from build123d import *

# Parameters (mm, degrees)
SKETCH1_W           = 120
SKETCH1_H           = 70
BOSS_EXTRUDE1_DEPTH = 50
SKETCH4_W           = 116
SKETCH4_H           = 66
CUT_EXTRUDE1_DEPTH  = 48
SKETCH5_R           = 4
SKETCH5_R_2         = 2.125
SKETCH5_R_3         = 3.805710372
BOSS_EXTRUDE2_DEPTH = 48
SKETCH7_R           = 4
SKETCH7_R_2         = 2.125
BOSS_EXTRUDE3_DEPTH = 8
SKETCH9_R           = 3
CUT_EXTRUDE2_DEPTH  = 3
CUT_EXTRUDE3_START  = -3
SKETCH10_R          = 3
CUT_EXTRUDE3_DEPTH  = 3


with BuildPart() as part:
    # Sketch1 → Boss-Extrude1 (new body)
    with BuildSketch(Plane(origin=(0, 0, 0), x_dir=(1, 0, 0), z_dir=(0, 1, 0))):
        Rectangle(SKETCH1_W, SKETCH1_H)
    extrude(amount=BOSS_EXTRUDE1_DEPTH)

    # Sketch4 → Cut-Extrude1 (cut)
    with BuildSketch(Plane(origin=(0, 50, 0), x_dir=(1, 0, 0), z_dir=(0, 1, 0))):
        Rectangle(SKETCH4_W, SKETCH4_H)
    extrude(amount=-CUT_EXTRUDE1_DEPTH, mode=Mode.SUBTRACT)

    # Sketch5 → Boss-Extrude2 (add)
    # profile 1 of 4: a face of its own
    with BuildSketch(Plane(origin=(0, 2, 0), x_dir=(1, 0, 0), z_dir=(0, 1, 0))):
        with Locations(Location((-53.5, 28.5, 0), (0, 0, 270))):
            Circle(SKETCH5_R)
        with Locations(Location((-53.5, 28.5, 0), (0, 0, 270))):
            Circle(SKETCH5_R_2, mode=Mode.SUBTRACT)
    # profile 2 of 4: a face of its own
    with BuildSketch(Plane(origin=(0, 2, 0), x_dir=(1, 0, 0), z_dir=(0, 1, 0))):
        with Locations(Location((-53.5, -28.5, 0), (0, 0, 270))):
            Circle(SKETCH5_R_3)
        with Locations(Location((-53.5, -28.5, 0), (0, 0, 270))):
            Circle(SKETCH5_R_2, mode=Mode.SUBTRACT)
    # profile 3 of 4: a face of its own
    with BuildSketch(Plane(origin=(0, 2, 0), x_dir=(1, 0, 0), z_dir=(0, 1, 0))):
        with Locations(Location((53.5, -28.5, 0), (0, 0, 270))):
            Circle(SKETCH5_R)
        with Locations(Location((53.5, -28.5, 0), (0, 0, 270))):
            Circle(SKETCH5_R_2, mode=Mode.SUBTRACT)
    # profile 4 of 4: a face of its own
    with BuildSketch(Plane(origin=(0, 2, 0), x_dir=(1, 0, 0), z_dir=(0, 1, 0))):
        with Locations(Location((53.5, 28.5, 0), (0, 0, 270))):
            Circle(SKETCH5_R)
        with Locations(Location((53.5, 28.5, 0), (0, 0, 270))):
            Circle(SKETCH5_R_2, mode=Mode.SUBTRACT)
    extrude(amount=BOSS_EXTRUDE2_DEPTH)

    # Sketch7 → Boss-Extrude3 (add)
    # profile 1 of 8: a face of its own
    with BuildSketch(Plane(origin=(0, 2, 0), x_dir=(1, 0, 0), z_dir=(0, 1, 0))):
        with Locations(Location((41.989163704, 23.984280939, 0), (0, 0, 270))):
            Circle(SKETCH7_R)
        with Locations(Location((41.989163704, 23.984280939, 0), (0, 0, 270))):
            Circle(SKETCH7_R_2, mode=Mode.SUBTRACT)
    # profile 2 of 8: a face of its own
    with BuildSketch(Plane(origin=(0, 2, 0), x_dir=(1, 0, 0), z_dir=(0, 1, 0))):
        with Locations(Location((27.989163704, 23.984280939, 0), (0, 0, 270))):
            Circle(SKETCH7_R)
        with Locations(Location((27.989163704, 23.984280939, 0), (0, 0, 270))):
            Circle(SKETCH7_R_2, mode=Mode.SUBTRACT)
    # profile 3 of 8: a face of its own
    with BuildSketch(Plane(origin=(0, 2, 0), x_dir=(1, 0, 0), z_dir=(0, 1, 0))):
        with Locations(Location((27.989163704, -25.015719061, 0), (0, 0, 270))):
            Circle(SKETCH7_R)
        with Locations(Location((27.989163704, -25.015719061, 0), (0, 0, 270))):
            Circle(SKETCH7_R_2, mode=Mode.SUBTRACT)
    # profile 4 of 8: a face of its own
    with BuildSketch(Plane(origin=(0, 2, 0), x_dir=(1, 0, 0), z_dir=(0, 1, 0))):
        with Locations(Location((41.989163704, -25.015719061, 0), (0, 0, 270))):
            Circle(SKETCH7_R)
        with Locations(Location((41.989163704, -25.015719061, 0), (0, 0, 270))):
            Circle(SKETCH7_R_2, mode=Mode.SUBTRACT)
    # profile 5 of 8: a face of its own
    with BuildSketch(Plane(origin=(0, 2, 0), x_dir=(1, 0, 0), z_dir=(0, 1, 0))):
        with Locations(Location((13.265207025, -17.861812849, 0), (0, 0, 270))):
            Circle(SKETCH7_R)
        with Locations(Location((13.265207025, -17.861812849, 0), (0, 0, 270))):
            Circle(SKETCH7_R_2, mode=Mode.SUBTRACT)
    # profile 6 of 8: a face of its own
    with BuildSketch(Plane(origin=(0, 2, 0), x_dir=(1, 0, 0), z_dir=(0, 1, 0))):
        with Locations(Location((13.265207025, 17.388187151, 0), (0, 0, 270))):
            Circle(SKETCH7_R)
        with Locations(Location((13.265207025, 17.388187151, 0), (0, 0, 270))):
            Circle(SKETCH7_R_2, mode=Mode.SUBTRACT)
    # profile 7 of 8: a face of its own
    with BuildSketch(Plane(origin=(0, 2, 0), x_dir=(1, 0, 0), z_dir=(0, 1, 0))):
        with Locations(Location((-46.734792975, 17.388187151, 0), (0, 0, 270))):
            Circle(SKETCH7_R)
        with Locations(Location((-46.734792975, 17.388187151, 0), (0, 0, 270))):
            Circle(SKETCH7_R_2, mode=Mode.SUBTRACT)
    # profile 8 of 8: a face of its own
    with BuildSketch(Plane(origin=(0, 2, 0), x_dir=(1, 0, 0), z_dir=(0, 1, 0))):
        with Locations(Location((-46.734792975, -17.861812849, 0), (0, 0, 270))):
            Circle(SKETCH7_R)
        with Locations(Location((-46.734792975, -17.861812849, 0), (0, 0, 270))):
            Circle(SKETCH7_R_2, mode=Mode.SUBTRACT)
    extrude(amount=BOSS_EXTRUDE3_DEPTH)

    # Sketch9 → Cut-Extrude2 (cut)
    with BuildSketch(Plane(origin=(60, 0, 0), x_dir=(0, 0, -1), z_dir=(1, 0, 0))):
        with Locations((0, 11.776029547)):
            Circle(SKETCH9_R)
    extrude(amount=-CUT_EXTRUDE2_DEPTH, mode=Mode.SUBTRACT)

    # Sketch10 → Cut-Extrude3 (cut)
    with BuildSketch(Plane.ZY.offset(60).offset(CUT_EXTRUDE3_START)):
        with Locations(Location((0, 11.776029547, 0), (0, 0, 180))):
            Circle(SKETCH10_R)
    extrude(amount=CUT_EXTRUDE3_DEPTH, mode=Mode.SUBTRACT)


solid = part.part
Verification items for the finished model (mm, model axes). A direction names the side the tool comes from. Round coordinates to 2 decimals unless told otherwise and drop trailing zeros. Loops run counter-clockwise (first coordinate to the right, second up) from the corner with the lowest first, then second, coordinate; pieces in that order, holes last. Notation, with made-up numbers: (-32.5, -25) - (-27.5, -25) arc R19 cw to (-27.5, -18) - close; hole circle Ø9 at (86, 76). An arc over 180 degrees is marked (long way). Use one line per item in the form item = value.
1. Section check C-C on x = -53.5. Record the cut outline in (y, z) (3 decimals), and give its area (3 significant figures).
A:
outline = (0, -35) - (50, -35) - (50, -33) - (2, -33) - (2, -32.5) - (50, -32.5) - (50, -30.625) - (2, -30.625) - (2, -26.375) - (50, -26.375) - (50, -24.5) - (2, -24.5) - (2, 24.694) - (50, 24.694) - (50, 26.375) - (2, 26.375) - (2, 30.625) - (50, 30.625) - (50, 32.306) - (2, 32.306) - (2, 33) - (50, 33) - (50, 35) - (0, 35) - close
area = 673 mm²
2. Section check B-B on z = 0. Record the cut outline in (x, y).
A:
outline = (-60, 0) - (60, 0) - (60, 8.78) - (58, 8.78) - (58, 2) - (-58, 2) - (-58, 8.78) - (-60, 8.78) - close; (-60, 14.78) - (-58, 14.78) - (-58, 50) - (-60, 50) - close; (58, 14.78) - (60, 14.78) - (60, 50) - (58, 50) - close
3. Scan lines: probe 1 along X at (y, z) = (18, -28.5) (3 decimals); probe 2 along X at (y, z) = (34, 28.5) (3 decimals); probe 3 along Z at (x, y) = (-28.5, 40). Record each from-to range of solid material in increasing order.
A:
probe_1 = -60 to -58, -57.5 to -55.625, -51.375 to -49.5, 49.5 to 51.375, 55.625 to 57.5, 58 to 60
probe_2 = -60 to -58, -57.306 to -55.625, -51.375 to -49.694, 49.5 to 51.375, 55.625 to 57.5, 58 to 60
probe_3 = -35 to -33, 33 to 35
4. Section check A-A on y = 22.5. Give the number of separate pieces and of enclosed holes in the cut face, and give its area (3 significant figures).
A:
separate_pieces = 5
enclosed_holes = 5
area = 884 mm²
5. Gauge pin test, flat ends, axial feed: pin 1 Ø4.5 at (x, z) = (14, 17) entering from +Y; pin 2 Ø1 at (x, z) = (39.5, -5.5) entering from +Y. Record the tip position at first contact, or that the pin passes through.
A:
pin_1 = 10
pin_2 = 2
6. Draft check along Z on faces 1 (the flat face through (60, 25, 0)), 2 (the cylindrical face through (13.36, 5.94, -19.51)). Enter one of: pulls with the +Z half, pulls with the -Z half, needs draft (parallel to the pull), parting line crosses it, or undercut.
A:
face_1 = needs draft
face_2 = undercut
7. Access from +Z, -Z, +X, -X, +Y, -Y to the whole of each face (thin tool, end or side, straight path). Record for faces 3 (the flat face through (51.8, 50, -26.8)), 4 (the cylindrical face through (14.467, 5.944, -13.573)).
A:
face_3 = +Z, -Z, +X, -X, +Y
face_4 = +Y
